Geometry: final body of the model. Coordinates: model frame, mm. A direction names the side the tool comes from. Give positions to 0.01 mm unless a question says otherwise; leave off trailing zeros. Order: outer loops, then holes, each group sorted by start corner. A loop starts at its lowest first (then second) coordinate and runs counter-clockwise, first axis right, second up. Notation, with made-up numbers: (38, 26) -> (55, 26) arc R19 cw to (55, 52) -> close; hole circle Ø10 at (65, -33.75). An arc over 180 degrees is marked (long way). Write item = value, one per line.
```python
from build123d import *

# Parameters (mm, degrees)
DODANIE_WYCI_GNI_CIE1_DEPTH = 197
DODANIE_WYCI_GNI_CIE2_DEPTH = 1.75
SZKIC3_R                    = 2.5
WYTNIJ_WYCI_GNI_CIE1_DEPTH  = 466
SZKIC4_R                    = 2.5
WYTNIJ_WYCI_GNI_CIE2_DEPTH  = 5
SZKIC5_R                    = 2.5
WYTNIJ_WYCI_GNI_CIE3_DEPTH  = 5


with BuildPart() as part:
    # Szkic1 → Dodanie-wyciągnięcie1 (new body, symmetric)
    with BuildSketch(Plane(origin=(0, 0, 0), x_dir=(1, 0, 0), z_dir=(0, 1, 0))):
        Polygon((-422.25, 0), (0, 0), (132, 132), (132, 153.2), (133.75, 153.2), (133.75, 131.275126266), (0.724873734, -1.75), (-424, -1.75), (-424, 0), (-424, 15), (-422.25, 15), align=None)
    extrude(amount=DODANIE_WYCI_GNI_CIE1_DEPTH, both=True)

    # Szkic2 → Dodanie-wyciągnięcie2 (add)
    with BuildSketch(Plane.XZ.offset(197)):
        Polygon((-422.25, -15), (-422.25, 0), (0, 0), (132, -132), (132, -153.213203436), (-6.213203436, -15), align=None)
    dodanie_wyci_gni_cie2 = extrude(amount=-DODANIE_WYCI_GNI_CIE2_DEPTH)

    # Lustro1: Dodanie-wyciągnięcie2 across plane
    add(dodanie_wyci_gni_cie2.mirror(Plane.ZX))

    # Szkic3 → Wytnij-wyciągnięcie1 (cut)
    with BuildSketch(Plane.XZ.offset(197)):
        with Locations((-414, -6.25)):
            Circle(SZKIC3_R)
        with Locations((-214, -6.25)):
            Circle(SZKIC3_R)
        with Locations((-14, -6.25)):
            Circle(SZKIC3_R)
        with Locations((122.221470087, -131.060304852)):
            Circle(SZKIC3_R)
    extrude(amount=-WYTNIJ_WYCI_GNI_CIE1_DEPTH, mode=Mode.SUBTRACT)

    # Szkic4 → Wytnij-wyciągnięcie2 (cut)
    with BuildSketch(Plane(origin=(133.75, 0, 0), x_dir=(0, 0, -1), z_dir=(1, 0, 0))):
        with Locations((139.275126266, 0)):
            Circle(SZKIC4_R)
    extrude(amount=-WYTNIJ_WYCI_GNI_CIE2_DEPTH, mode=Mode.SUBTRACT)

    # Szkic5 → Wytnij-wyciągnięcie3 (cut)
    with BuildSketch(Plane.ZY.offset(424)):
        with Locations((-6.25, 0)):
            Circle(SZKIC5_R)
    extrude(amount=-WYTNIJ_WYCI_GNI_CIE3_DEPTH, mode=Mode.SUBTRACT)


solid = part.part
```
1) First-contact query: P1, Ø6.5, axis at y = 64.5, z = -141.5, coming from the -X side; P2, Ø12, axis at y = -56.5, z = -10.5, coming from the +X side; P3, Ø8, axis at y = -133.5, z = -100.5, coming from the -X side. Flat tips, straight axial feed; report the tip coordinate or a pass-through.
Check sheet entries:
P1 = 132
P2 = 18.97
P3 = 96.5
2) Section query A-A (x = -137). Output: boundary loops of the cut face in (y, z), plus the area to 3 significant figures.
Check sheet entries:
outline = (-197, -15) -> (-195.25, -15) -> (-195.25, 0) -> (195.25, 0) -> (195.25, -15) -> (197, -15) -> (197, 1.75) -> (-197, 1.75) -> close
area = 742 mm²
3) Line query: line 1 (Z direction, x = -356, y = -179.5); line 2 (Z direction, x = -214, y = -195.7); line 3 (X direction, y = -169, z = -8). Output: solid intervals per line, ascending. Write a range as from..to.
Check sheet entries:
line_1 = 0..1.75
line_2 = -15..-8.75, -3.75..1.75
line_3 = -424..-422.25, 8..10.47
4) Reachability of faces 4 (the face through (-422.25, 3, -8)), 5 (the face through (68.169, 2.758, -65.694)), 6 (the face through (132, 3, -142)) from +Z, -Z, +X, -X, +Y, -Y: full face, straight path, thin tool, end or side. Return the list, or none.
Check sheet entries:
face_4 = -Z
face_5 = +Z, +X, +Y, -Y
face_6 = -Z, -X
5) Section query B-B (z = -73). Output: boundary loops of the cut face in (x, y).
Check sheet entries:
outline = (51.79, -197) -> (75.47, -197) -> (75.47, 197) -> (51.79, 197) -> (51.79, 195.25) -> (73, 195.25) -> (73, -195.25) -> (51.79, -195.25) -> close
6) Section query C-C (y = -125). Output: boundary loops of the cut face in (x, z), plus the area to 3 significant figures.
Check sheet entries:
outline = (-424, -15) -> (-422.25, -15) -> (-422.25, 0) -> (0, 0) -> (132, -132) -> (132, -153.2) -> (133.75, -153.2) -> (133.75, -131.28) -> (0.72, 1.75) -> (-424, 1.75) -> close
area = 1,130 mm²
7) Mould query, pull axis Y, two halves, no side actions, for faces 1 (the face through (-123, 197, -12)), 2 (the face through (-209, 3, 1.75)), 3 (the face through (-144, 195.25, -14)). Classes: +Y half, -Y half, draft (parallel to the pull), parting line (faces both ways), or undercut.
Check sheet entries:
face_1 = +Y half
face_2 = draft
face_3 = undercut
